from build123d import *

# Parameters (mm, degrees)
BOSS_EXTRUDE1_DEPTH = 6.35


with BuildPart() as part:
    # Sketch2 → Boss-Extrude1 (new body)
    with BuildSketch(Plane(origin=(0, 0, 0), x_dir=(0, 0, -1), z_dir=(1, 0, 0))):
        Polygon((-152.4, 101.6), (152.4, 101.6), (152.4, 88.9), (158.75, 88.9), (158.75, 69.85), (152.4, 69.85), (152.4, 50.8), (158.75, 50.8), (158.75, 31.75), (152.4, 31.75), (152.4, 12.7), (158.75, 12.7), (158.75, 0), (139.7, 0), (139.7, 6.35), (114.3, 6.35), (114.3, 0), (88.9, 0), (88.9, 6.35), (63.5, 6.35), (63.5, 0), (38.1, 0), (38.1, 6.35), (12.7, 6.35), (12.7, 0), (-12.7, 0), (-12.7, 6.35), (-38.1, 6.35), (-38.1, 0), (-63.5, 0), (-63.5, 6.35), (-88.9, 6.35), (-88.9, 0), (-114.3, 0), (-114.3, 6.35), (-139.7, 6.35), (-139.7, 0), (-158.75, 0), (-158.75, 12.7), (-152.4, 12.7), (-152.4, 31.75), (-158.75, 31.75), (-158.75, 50.8), (-152.4, 50.8), (-152.4, 69.85), (-158.75, 69.85), (-158.75, 88.9), (-152.4, 88.9), align=None)
        with BuildLine():
            Line((-76.2, 50.8), (76.2, 50.8))
            ThreePointArc((76.2, 50.8), (88.9, 63.5), (76.2, 76.2))
            Line((76.2, 76.2), (-76.2, 76.2))
            ThreePointArc((-76.2, 76.2), (-88.9, 63.5), (-76.2, 50.8))
        make_face(mode=Mode.SUBTRACT)
    extrude(amount=BOSS_EXTRUDE1_DEPTH)


solid = part.part
Read the model definition and answer for the solid it produces. Units are mm, in the model's axes. A direction names the side the tool comes from. Give positions to 0.01 mm unless a question says otherwise; leave off trailing zeros. Loops run counter-clockwise (first coordinate to the right, second up) from the corner with the lowest first, then second, coordinate; pieces in that order, holes last. Notation, with made-up numbers: (11.25, 77.25) - (43.25, 77.25) arc R28 cw to (43.25, 103.25) - close; hole circle Ø8 at (14, 75). An arc over 180 degrees is marked (long way). Answer as CSV lines item,"result". Start each with the question number.
1) Find section C-C (z = 137). Write down the section's boundary in (x, y).
2) Find section A-A (z = -33). Write down the section's boundary in (x, y), then the cut area to 3 significant figures.
3) Which of the six approach directions +Z, -Z, +X, -X, +Y, -Y give full straight-line access (tool end or side, diameter ignored) to faces 1 (the face through (3, 6.35, 127)), 2 (the face through (3, 69.85, -156)), 3 (the face through (3.131, 63.221, -88.897))?
4) Determine the mould class of faces 4 (the face through (3, 3, 63.5)), 5 (the face through (3, 6.35, -127)), 6 (the face through (3, 101.6, 2)), 7 (the face through (3, 31.75, -156)) for opening direction Y: released by +Y, released by -Y, zero draft, split by the parting line, or undercut.
5) Each of these flat-tipped pins is pushed along its axis until it touches: pin 1 Ø1.9 at (x, z) = (4.5, -157) entering from +Y; pin 2 Ø1.9 at (x, z) = (3.5, 22.5) entering from -Y; pin 3 Ø3 at (x, y) = (2.5, 96) entering from -Z. Where does it stop, or does it pass through?
6) Find section B-B (z = 79). Write down the section's boundary in (x, y).
7) Straight lines are drawn through the part: L1, parallel to Y at x = 1.25, z = 1; L2, parallel to Y at x = 3.5, z = 23; L3, parallel to Z at x = 1.25, y = 64.5. For each, find the intervals that lie inside material, in ascending order. Write a range as from..to.
Findings below:
1,outline,"(0, 6.35) - (6.35, 6.35) - (6.35, 101.6) - (0, 101.6) - close"
2,outline,"(0, 6.35) - (6.35, 6.35) - (6.35, 50.8) - (0, 50.8) - close; (0, 76.2) - (6.35, 76.2) - (6.35, 101.6) - (0, 101.6) - close"
2,area,"444 mm^2"
3,face 1,"+X, -X, -Y"
3,face 2,"-Z, +X, -X"
3,face 3,"+X, -X"
4,face 4,"zero draft"
4,face 5,"released by -Y"
4,face 6,"released by +Y"
4,face 7,"undercut"
5,pin 1,"y = 88.9"
5,pin 2,"y = 6.35"
5,pin 3,"z = -152.4"
6,outline,"(0, 6.35) - (6.35, 6.35) - (6.35, 51.11) - (0, 51.11) - close; (0, 75.89) - (6.35, 75.89) - (6.35, 101.6) - (0, 101.6) - close"
7,L1,"0..50.8, 76.2..101.6"
7,L2,"6.35..50.8, 76.2..101.6"
7,L3,"-152.4..-88.86, 88.86..152.4"
